from build123d import *

# Parameters (mm, degrees)
F0_R     = 52.168743
F1_DEPTH = 3
F3_D     = 3
F7_D     = 3


with BuildPart() as f1:
    # F0 (on Top) → F1 (new body)
    with BuildSketch(Plane.XY):
        Circle(F0_R)
    extrude(amount=F1_DEPTH)

    # F3 (through all)
    with Locations(Plane(origin=(0, 0, 0), x_dir=(1, 0, 0), z_dir=(0, 0, -1))):
        with Locations((-14.456525, -16.74062), (9.536847, -16.74062)):
            Hole(F3_D / 2)

    # F4: F1 across plane


with BuildPart() as f1_1:
    add(f1.part)
    add(f1.part.mirror(Plane.XZ))

    # F7 (through all)
    with Locations(Plane.XY.offset(3)):
        with Locations((-29.232398, 21.0049), (-29.232398, -19.615047), (29.403359, 19.193865), (29.403359, -18.989682)):
            Hole(F7_D / 2)


solid = f1_1.part
Build history of the part. All positions in model axes, mm. Round coordinates to 2 decimals unless told otherwise and drop trailing zeros. Loops run counter-clockwise (first coordinate to the right, second up) from the corner with the lowest first, then second, coordinate; pieces in that order, holes last. Notation, with made-up numbers: (26, 87.25) -> (76, 87.25) arc R23 ccw to (76, 107.25) -> close; hole circle Ø2 at (28, -38). An arc over 180 degrees is marked (long way). Answer in a Markdown table with one row per item.
Item 1: Drill centre lines: L1, parallel to Y at x = 1, z = 1.95; L2, parallel to Y at x = 29, z = 1.15; L3, parallel to X at y = 21, z = 1.1. Where is each one in solid material? Low to high. Write a range as [from, to].
Answers below:
| item | result |
|---|---|
| L1 | y = [-52.16, 52.16] |
| L2 | y = [-43.37, -20.43], [-17.54, 17.75], [20.64, 43.37] |
| L3 | x = [-47.76, -30.73], [-27.73, 47.76] |
Item 2: Saw through at B-B (x = 11.5). Write the cut outline in (y, z), and give its area (3 significant figures).
Answers below:
| item | result |
|---|---|
| outline | (-50.89, 0) -> (50.89, 0) -> (50.89, 3) -> (-50.89, 3) -> close |
| area | 305 mm² |
Item 3: Saw through at C-C (y = 35). Write the cut outline in (x, z), and give its area (3 significant figures).
Answers below:
| item | result |
|---|---|
| outline | (-38.69, 0) -> (38.69, 0) -> (38.69, 3) -> (-38.69, 3) -> close |
| area | 232 mm² |
Item 4: Pin check, flat tip, straight feed: pin 1 (2.5 mm diameter, centred on x = 29.4, y = -18.99, fed in from -Z). Stop position of the tip, or through.
Answers below:
| item | result |
|---|---|
| pin 1 | passes through |
Item 5: Saw through at A-A (z = 1). Write the cut outline in (x, y), and give its area (3 significant figures).
Answers below:
| item | result |
|---|---|
| outline | circle Ø104.34 at (0, 0); hole circle Ø3 at (-29.23, -19.62); hole circle Ø3 at (-29.23, 21); hole circle Ø3 at (29.4, -18.99); hole circle Ø3 at (29.4, 19.19) |
| area | 8,520 mm² |
Item 6: Mould opens along Y. For faces 1 (the cylindrical face through (49.76, 15.67, 1.48)), 2 (the cylindrical face through (27.973, -18.539, 1.479)), 3 (the cylindrical face through (28.018, 18.619, 1.479)), 4 (the flat face through (-1, 1, 0)) say: +Y half, -Y half, draft (parallel to the pull), parting line (faces both ways), or undercut.
Answers below:
| item | result |
|---|---|
| face 1 | parting line |
| face 2 | undercut |
| face 3 | undercut |
| face 4 | draft |
